from build123d import *

# Parameters (mm, degrees)
CUT_EXTRUDE1_START = -2
CUT_EXTRUDE1_DEPTH = 2
CUT_EXTRUDE2_DEPTH = 11


with BuildPart() as part:
    # Sketch1 → Revolve1 (revolve)
    with BuildSketch(Plane.XY, mode=Mode.PRIVATE) as revolve1_sk:
        Polygon((0, 0), (7, 0), (7, 2), (11.5, 2), (11.5, 5), (9.5, 5), (9.5, 7), (0, 7), align=None)
    revolve(revolve1_sk.sketch.rotate(Axis((0, 7, 0), (0, -1, 0)), 90), axis=Axis((0, 7, 0), (0, -1, 0)))

    # Sketch3 → Cut-Extrude1 (cut)
    with BuildSketch(Plane.XZ.offset(CUT_EXTRUDE1_START)):
        with BuildLine():
            Line((0, 3.5), (6.062177826, 3.5))
            ThreePointArc((6.062177826, 3.5), (7, 0), (6.062177826, -3.5))
            Line((6.062177826, -3.5), (0, -3.5))
            ThreePointArc((0, -3.5), (-3.5, 0), (0, 3.5))
        make_face()
    extrude(amount=CUT_EXTRUDE1_DEPTH, mode=Mode.SUBTRACT)

    # Sketch4 → Cut-Extrude2 (cut)
    with BuildSketch(Plane(origin=(0, 7, 0), x_dir=(1, 0, 0), z_dir=(0, 1, 0))):
        with BuildLine():
            Line((0, 2.75), (11.166355717, 2.75))
            ThreePointArc((11.166355717, 2.75), (11.5, 0), (11.166355717, -2.75))
            Line((11.166355717, -2.75), (0, -2.75))
            ThreePointArc((0, -2.75), (-2.75, 0), (0, 2.75))
        make_face()
    extrude(amount=-CUT_EXTRUDE2_DEPTH, mode=Mode.SUBTRACT)


solid = part.part
Build history of the part. All positions in model axes, mm. A direction names the side the tool comes from. Round coordinates to 2 decimals unless told otherwise and drop trailing zeros. Write each loop counter-clockwise with the first axis right and the second up, starting at its lowest first coordinate (ties: lowest second). Pieces come first, ordered by that corner, then holes. Notation, with made-up numbers: M 54.25,70.25 L 102.25,70.25 A11 cw 102.25,78.25 Z; hole C 52.25,-17 d9. An arc over 180 degrees is marked long. Use CSV: the item, a comma, the result in double quotes.
1. Wall check: probe 1 along Z at (x, y) = (6.5, 5.5); probe 2 along Z at (x, y) = (-1.5, 6); probe 3 along X at (y, z) = (1, 1.25). Give the ranges that are in metal, low to high. Write a range as from..to.
Reply:
probe 1,"z = -6.93..-2.75, 2.75..6.93"
probe 2,"z = -9.38..-2.3, 2.3..9.38"
probe 3,"x = -6.89..-3.27"
2. Saw through at C-C (x = -8.5). Give the cut face in (y, z).
Reply:
outline,"M 2,-7.75 L 5,-7.75 L 5,-4.24 L 7,-4.24 L 7,4.24 L 5,4.24 L 5,7.75 L 2,7.75 Z"
3. Saw through at A-A (x = 9.5). Give the cut face in (y, z).
Reply:
outline,"M 2,-6.48 L 5,-6.48 L 5,-2.75 L 2,-2.75 Z; M 2,2.75 L 5,2.75 L 5,6.48 L 2,6.48 Z"
4. Two-plate mould, pull along Z, no slides. Class faces 1 (the face through (-11.49, 3.52, 0.47)), 2 (the face through (-2.4, 7, 2)), 3 (the face through (3, 1, 3.5)): +Z half, -Z half, draft (parallel to the pull), parting line (faces both ways), or undercut.
Reply:
face 1,"parting line"
face 2,"draft"
face 3,"undercut"
5. Saw through at B-B (z = 0). Give the cut face in (x, y), plus the area to 4 significant figures.
Reply:
outline,"M -11.5,2 L -7,2 L -7,0 L -3.5,0 L -3.5,2 L -2.75,2 L -2.75,7 L -9.5,7 L -9.5,5 L -11.5,5 Z"
area,"46.75 mm²"
6. Saw through at D-D (x = -2.25). Give the cut face in (y, z), plus the area to 3 significant figures.
Reply:
outline,"M 0,-6.63 L 2,-6.63 L 2,-11.28 L 5,-11.28 L 5,-9.23 L 7,-9.23 L 7,-1.58 L 2,-1.58 L 2,-2.68 L 0,-2.68 Z; M 0,2.68 L 2,2.68 L 2,1.58 L 7,1.58 L 7,9.23 L 5,9.23 L 5,11.28 L 2,11.28 L 2,6.63 L 0,6.63 Z"
area,"105 mm²"
7. Flat gauge pins, fed straight in: pin 1 (3 mm diameter, centred on y = 5.5, z = -8, fed in from +X); pin 2 (1 mm diameter, centred on x = 7, z = 8, fed in from -Y); pin 3 (1.5 mm diameter, centred on x = 5, z = -2.5, fed in from +Y); pin 4 (4 mm diameter, centred on x = 7, y = 5.5, fed in from +Z). Where does each tip first touch, or does it go through?
Reply:
pin 1,"stops at x = 9.43"
pin 2,"stops at y = 2"
pin 3,"stops at y = 7"
pin 4,"stops at z = 10.33"
8. Tool access for faces 4 (the face through (6, 5, 2.75)), 5 (the face through (-9.5, 5, 2.5)), 6 (the face through (-3.5, 0, -1.5)), 7 (the face through (3, 1, -3.5)), 8 (the face through (-7, 1, 0)): list every direction of +Z, -Z, +X, -X, +Y, -Y with a clear straight run to the whole face (end or side of a thin tool).
Reply:
face 4,"+X, +Y, -Y"
face 5,"+Y"
face 6,"+Z, -Z, +X, -X, -Y"
face 7,"+X, -Y"
face 8,"-Y"
